Check sheet for the modelled part. Datum: model origin and axes. Units: mm. A direction names the side the tool comes from. Round coordinates to 2 decimals unless told otherwise and drop trailing zeros. Loops run counter-clockwise (first coordinate to the right, second up) from the corner with the lowest first, then second, coordinate; pieces in that order, holes last. Notation, with made-up numbers: (33, 39) - (88, 39) arc R8 ccw to (88, 43) - close; hole circle Ø9 at (50.5, 32). An arc over 180 degrees is marked (long way). Return JSON: item names as keys, results as strings.
Solid Edge part; units mm, degrees
sketch "Sketch1" plane through (0, 0, 0) normal (0, -1, 0) x (1, 0, 0)
  line L0 (-63.5, 12.7) -> (63.5, 12.7)
  line L1 (63.5, -12.7) -> (63.5, 12.7)
  line L2 (38.1, -12.7) -> (63.5, -12.7)
  line L3 (50.8, 0) -> (38.1, -12.7)
  line L4 (0, 0) -> (50.8, 0)
  line L5 (0, 0) -> (-50.8, 0)
  line L6 (-50.8, 0) -> (-38.1, -12.7)
  line L7 (-38.1, -12.7) -> (-63.5, -12.7)
  line L8 (-63.5, -12.7) -> (-63.5, 12.7)
extrude "Protrusion1" add sketch "Sketch1" against normal blind 254
sketch "Sketch2" plane through (0, 0, 0) normal (0, -1, 0) x (1, 0, 0)
  circle A0 centre (0, -6.35) radius 19.05
extrude "ExtrudedProtrusion_2" add sketch "Sketch2" along normal blind 12.7
chamfer "Chamfer_1" distance 6.35 angle 45 1 edges at (-19.05, -12.7, -6.35)
sketch "Sketch3" plane through (0, 0, 0) normal (0, -1, 0) x (1, 0, 0)
  circle A0 centre (0, -6.35) radius 3.175
extrude "ExtrudedProtrusion_3" add sketch "Sketch3" against normal blind 241.3
sketch "Sketch4" plane through (0, 127, 12.7) normal (0, 0, 1) x (0, 1, 0)
  circle A0 centre (-76.2, 0) radius 12.7
extrude "ExtrudedProtrusion_6" add sketch "Sketch4" along normal blind 6.35
Q1. Depth check by flat-ended pin: P1, Ø12.5, axis at x = 1.5, z = -9.5, coming from the +Y side; P2, Ø4, axis at x = 11, y = 72, coming from the -Z side; P3, Ø1, axis at x = 40, y = 202.5, coming from the +Z side. Enter the tip coordinate at first touch or a pass-through.
Answer key:
{"P1": "stops at y = 241.3", "P2": "stops at z = 0", "P3": "stops at z = 12.7"}
Q2. Sectioned sample at C-C (y = 19). Enter the section's corners in (x, z) (3 decimals), plus the area to 3 significant figures.
Answer key:
{"outline": "(-63.5, -12.7) - (-38.1, -12.7) - (-50.8, 0) - (50.8, 0) - (38.1, -12.7) - (63.5, -12.7) - (63.5, 12.7) - (-63.5, 12.7) - close; circle Ø6.35 at (0, -6.35)", "area": "2,130 mm²"}
Q3. Sectioned sample at B-B (x = 48). Enter the section's corners in (y, z), plus the area to 3 significant figures.
Answer key:
{"outline": "(0, -12.7) - (254, -12.7) - (254, -2.8) - (0, -2.8) - close; (0, 0) - (254, 0) - (254, 12.7) - (0, 12.7) - close", "area": "5,740 mm²"}
Q4. Sectioned sample at D-D (y = 51). Enter the section's corners in (x, z) (3 decimals).
Answer key:
{"outline": "(-63.5, -12.7) - (-38.1, -12.7) - (-50.8, 0) - (50.8, 0) - (38.1, -12.7) - (63.5, -12.7) - (63.5, 12.7) - (12.698, 12.7) - (12.698, 19.05) - (-12.698, 19.05) - (-12.698, 12.7) - (-63.5, 12.7) - close; circle Ø6.35 at (0, -6.35)"}
Q5. Draft check along Z on faces 1 (the face through (-2.84, -12.3, 6.44)), 2 (the face through (-44.5, 125.2, -6.3)), 3 (the face through (46, 0, 3)). Enter one of: released by +Z, released by -Z, zero draft, split by the parting line, or undercut.
Answer key:
{"face 1": "split by the parting line", "face 2": "undercut", "face 3": "zero draft"}
Q6. Sectioned sample at A-A (z = -6.35). Enter the section's corners in (x, y) (3 decimals), plus the area to 3 significant figures.
Answer key:
{"outline": "(-63.5, 0) - (-44.45, 0) - (-44.45, 254) - (-63.5, 254) - close; (-19.05, -6.35) - (-12.7, -12.7) - (12.7, -12.7) - (19.05, -6.35) - (19.05, 0) - (3.175, 0) - (3.175, 241.3) - (-3.175, 241.3) - (-3.175, 0) - (-19.05, 0) - close; (44.45, 0) - (63.5, 0) - (63.5, 254) - (44.45, 254) - close", "area": "11,700 mm²"}
Q7. Tool access check on faces 4 (the face through (44.5, 125.2, -6.3)), 5 (the face through (-0.69, 118.96, -9.45)), 6 (the face through (-2.48, -3.131, -25.238)), 7 (the face through (0.558, 38.112, 15.831)), 8 (the face through (0, 241.3, -6)). Record the directions out of +Z, -Z, +X, -X, +Y, -Y that give a thin tool (end or side, any length) a straight path to the whole face; none if there is none.
Answer key:
{"face 4": "+Y, -Y", "face 5": "+Y", "face 6": "-Y", "face 7": "+Z", "face 8": "-Z, +Y"}
Q8. Scan lines: probe 1 along Y at (x, z) = (0, 15); probe 2 along X at (y, z) = (31.5, -4.5); probe 3 along Z at (x, y) = (-36.5, 210.5). Record each from-to range of solid material in increasing order. Write a range as [from, to].
Answer key:
{"probe 1": "y = [38.1, 63.5]", "probe 2": "x = [-63.5, -46.3], [-2.58, 2.58], [46.3, 63.5]", "probe 3": "z = [0, 12.7]"}
